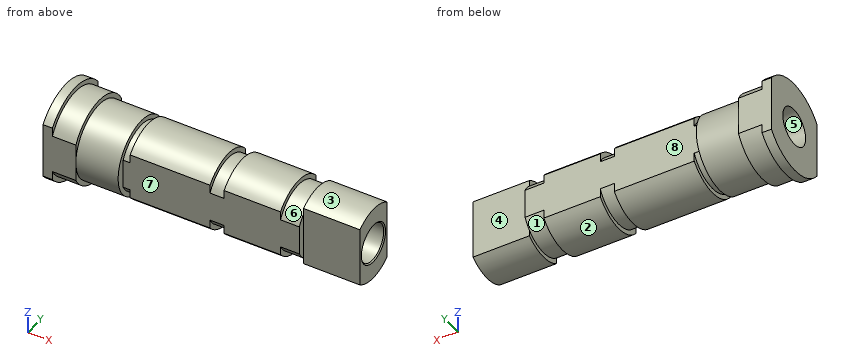
Autodesk Inventor part; units mm, degrees
ref_plane "YZ Plane" through (0, 0, 0) normal (1, 0, 0) x (0, 1, 0)
ref_plane "XZ Plane" through (0, 0, 0) normal (0, 1, 0) x (-1, 0, 0)
ref_plane "XY Plane" through (0, 0, 0) normal (0, 0, 1) x (1, 0, 0)
sketch "Sketch1" plane through (0, 0, 0) normal (0, 0, 1) x (1, 0, 0)
  line L0 (0, 0) -> (1, 0)
  line L1 (1, 0) -> (1, 5)
  line L2 (1, 5) -> (0, 5)
  line L3 (0, 5) -> (0, 0)
  line L4 (1, 0) -> (3.5, 0)
  line L5 (3.5, 0) -> (3.5, 4.5)
  line L6 (3.5, 4.5) -> (1, 4.5)
  line L7 (1, 4.5) -> (1, 0)
  line L8 (8.75, 0) -> (17.25, 0)
  line L9 (17.25, 0) -> (17.25, 4)
  line L10 (17.25, 4) -> (8.75, 4)
  line L11 (8.75, 4) -> (8.75, 0)
  line L12 (17.25, 0) -> (18.75, 0)
  line L13 (18.75, 0) -> (18.75, 3.5)
  line L14 (18.75, 3.5) -> (17.25, 3.5)
  line L15 (17.25, 3.5) -> (17.25, 0)
  line L16 (18.75, 0) -> (24.75, 0)
  line L17 (24.75, 0) -> (24.75, 4)
  line L18 (24.75, 4) -> (18.75, 4)
  line L19 (18.75, 4) -> (18.75, 0)
  line L20 (24.75, 0) -> (26.75, 0)
  line L21 (26.75, 0) -> (26.75, 3.5)
  line L22 (26.75, 3.5) -> (24.75, 3.5)
  line L23 (24.75, 3.5) -> (24.75, 0)
  line L24 (26.75, 0) -> (32.75, 0)
  line L25 (32.75, 0) -> (32.75, 4)
  line L26 (32.75, 4) -> (26.75, 4)
  line L27 (26.75, 4) -> (26.75, 0)
  line L28 (3.5, 0) -> (8, 0)
  line L29 (8, 0) -> (8, 4)
  line L30 (8, 4) -> (3.5, 4)
  line L31 (3.5, 4) -> (3.5, 0)
  line L32 (8, 0) -> (8.75, 0)
  line L33 (8.75, 0) -> (8.75, 3.5)
  line L34 (8.75, 3.5) -> (8, 3.5)
  line L35 (8, 3.5) -> (8, 0)
  dimension "d0" = 1
  dimension "d1" = 3.5
  dimension "d2" = 32.75
  dimension "d3" = 2
  dimension "d5" = 24.75
  dimension "d6" = 1.5
  dimension "d7" = 17.25
  dimension "d9" = 8
  dimension "d10" = 0.75
  dimension "d11" = 8
  dimension "d12" = 7
  dimension "d13" = 10
  dimension "d14" = 9
  dimension "d15" = 8
revolve "Revolution1" add sketch "Sketch1" angle 360 about axis through (1, 0, 0) along (1, 0, 0)
thread "Thread1"
thread "Thread2"
sketch "Sketch2" plane through (0, 0, 0) normal (0, 0, 1) x (1, 0, 0)
  line L0 (32.75, 2.375) -> (26.75, 2.375)
  line L1 (26.75, 2.375) -> (26.75, 3.125)
  line L2 (26.75, 3.125) -> (8, 3.125)
  line L3 (8, 3.125) -> (8, 5)
  line L4 (8, 5) -> (32.75, 5)
  line L5 (32.75, 5) -> (32.75, 2.375)
  line L6 (0, 4) -> (4, 4)
  line L7 (4, 4) -> (4, 5)
  line L8 (4, 5) -> (0, 5)
  line L9 (0, 5) -> (0, 4)
  point P0 (0, 0)
  dimension "d21" = 4
  dimension "d22" = 4
  dimension "d23" = 1
  dimension "d24" = 2.375
  dimension "d25" = 32.75
  dimension "d26" = 3.125
  dimension "d27" = 8
  dimension "d28" = 26.75
extrude "Extrusion1" cut sketch "Sketch2" along normal mid plane 10
mirror "Mirror1" about plane through (0, 0, 0) normal (0, 1, 0) of "Extrusion1"
hole "Hole1" at (0, 0, 0) direction (1, 0, 0) diameter 4 end through all
chamfer "Chamfer1" distance 0.125 angle 45 1 edges at (32.75, 0, -2)
properties part number "404-01" material "Brass, Soft Yellow"
Can you work these out from the model? Positions are in its coordinate system, mm. Face numbers are marked on the shaded views. A direction names the side the tool comes from. Round coordinates to 2 decimals unless told otherwise and drop trailing zeros. Loops run counter-clockwise (first coordinate to the right, second up) from the corner with the lowest first, then second, coordinate; pieces in that order, holes last. Notation, with made-up numbers: M 84,18.5 L 121,18.5 A23 ccw 121,40.5 Z; hole C -25,35.25 d3. An arc over 180 degrees is marked long. Answer as a JSON object with one key per item and string values. Group by question number.
Q1. On a 3-axis mill with a long thin cutter (end or side, diameter ignored), from which of +Z, -Z, +X, -X, +Y, -Y can I reach the whole of each face in a straight line? I mean the marked faces 1, 2, 3 and 4. Say none if no direction works.
Q2. Please list where these lines run through material, in increasing order: L1, parallel to Z at x = 20.5, y = 0; L2, parallel to X at y = 2.25, z = 3.25; L3, parallel to Y at x = 24, z = 0 (3 decimals).
Q3. Imagine slicing it at C-C, the plane x = 3. Please give me the cut outline in (y, z).
Q4. Will these pins go through, and if not, where does the flat tip stop? pin 1 (2 mm diameter, centred on x = 15.5, y = 0, fed in from +Z); pin 2 (3 mm diameter, centred on x = 29.5, z = 0.5, fed in from -Y) (3 decimals); pin 3 (2 mm diameter, centred on x = 6, z = 2.5, fed in from +Y).
Q5. Imagine slicing it at D-D, the plane x = 7. Please give me the cut outline in (y, z).
Q6. Imagine slicing it at A-A, the plane x = 14. Please give me the cut outline in (y, z) (3 decimals).
Q7. We'd pull the mould along Y, two halves only. Please class the marked faces 5, 6, 7 and 8: +Y half, -Y half, draft (parallel to the pull), parting line (faces both ways), or undercut.
Findings:
{
 "1": {"face 1": "-Z", "face 2": "-Z, +X", "face 3": "+Z, +X", "face 4": "+Z, -Z, +X, +Y"},
 "2": {"L1": "z = -4 to -2, 2 to 4", "L2": "x = 0 to 8, 8.75 to 17.25, 18.75 to 24.75, 26.75 to 32.75", "L3": "y = -3.125 to -2, 2 to 3.125"},
 "3": {"outline": "M -4,-2.06 A4.5 ccw 4,-2.06 L 4,2.06 A4.5 ccw -4,2.06 Z; hole C 0,0 d4"},
 "4": {"pin 1": "stops at z = 4", "pin 2": "stops at y = -2.375", "pin 3": "stops at y = 3.71"},
 "5": {"outline": "C 0,0 d8; hole C 0,0 d4"},
 "6": {"outline": "M -3.125,-2.497 A4 ccw 3.125,-2.497 L 3.125,2.497 A4 ccw -3.125,2.497 Z; hole C 0,0 d4"},
 "7": {"face 5": "undercut", "face 6": "parting line", "face 7": "-Y half", "face 8": "+Y half"}
}
